Could you check a few things on this model? Use its own coordinates, in mm. Face numbers are marked on the shaded views. A direction names the side the tool comes from. Round coordinates to 2 decimals unless told otherwise and drop trailing zeros. Write each loop counter-clockwise with the first axis right and the second up, starting at its lowest first coordinate (ties: lowest second). Pieces come first, ordered by that corner, then holes. Notation, with made-up numbers: M 7.25,14 L 52.25,14 A20 ccw 52.25,51 Z; hole C -26,-4.5 d10. An arc over 180 degrees is marked long. One line per question, with ' | ' between items. Start each with the question number.
```python
from build123d import *

# Parameters (mm, degrees)
SKETCH4_R           = 3.175
SKETCH4_R_2         = 3.96875
SKETCH4_R_3         = 5.1
SKETCH4_R_4         = 1.6
SKETCH4_R_5         = 2
BOSS_EXTRUDE2_DEPTH = 6.35


with BuildPart() as part:
    # Sketch4 → Boss-Extrude2 (new body)
    with BuildSketch(Plane(origin=(0, 0, 0), x_dir=(1, 0, 0), z_dir=(0, 1, 0))):
        with BuildLine():
            Line((40.257702493, -18.4375), (21.46596982, -18.4375))
            ThreePointArc((21.46596982, -18.4375), (19.855794242, -18.080532669), (18.547340491, -17.076520793))
            Line((18.547340491, -17.076520793), (9.268629328, -6.01858343))
            ThreePointArc((9.268629328, -6.01858343), (6.86044471, -4.691952465), (4.186444468, -5.331503545))
            Line((4.186444468, -5.331503545), (-15.327970397, -18.794247435))
            ThreePointArc((-15.327970397, -18.794247435), (-21.058470009, -18.050117151), (-20.917416467, -12.27322702))
            Line((-20.917416467, -12.27322702), (-8.5725, 0.781747009))
            Line((-8.5725, 0.781747009), (-8.5725, 26.9875))
            ThreePointArc((-8.5725, 26.9875), (-7.456576836, 29.681576836), (-4.7625, 30.7975))
            Line((-4.7625, 30.7975), (52.3875, 30.7975))
            ThreePointArc((52.3875, 30.7975), (55.081576836, 29.681576836), (56.1975, 26.9875))
            Line((56.1975, 26.9875), (56.1975, 19.362095927))
            ThreePointArc((56.1975, 19.362095927), (55.797199918, 17.662082259), (54.680415238, 16.319294633))
            Line((54.680415238, 16.319294633), (48.985566477, 12.027918285))
            ThreePointArc((48.985566477, 12.027918285), (47.868781798, 10.685130659), (47.468481715, 8.985116992))
            Line((47.468481715, 8.985116992), (47.468481715, -10.980610773))
            ThreePointArc((47.468481715, -10.980610773), (47.203372649, -12.376980446), (46.444939319, -13.579024524))
            Line((46.444939319, -13.579024524), (43.044160097, -17.225913752))
            ThreePointArc((43.044160097, -17.225913752), (41.776936446, -18.121498883), (40.257702493, -18.4375))
        make_face()
        with Locations(Location((0, 0, 0), (0, 0, 270))):
            Circle(SKETCH4_R, mode=Mode.SUBTRACT)
        with Locations(Location((-1.5875, 21.9075, 0), (0, 0, 270))):
            Circle(SKETCH4_R_2, mode=Mode.SUBTRACT)
        with Locations(Location((49.2125, 21.9075, 0), (0, 0, 270))):
            Circle(SKETCH4_R_2, mode=Mode.SUBTRACT)
        with Locations(Location((39.848481715, -4.1275, 0), (0, 0, 270))):
            Circle(SKETCH4_R_3, mode=Mode.SUBTRACT)
        with Locations(Location((39.848481715, -14.6275, 0), (0, 0, 270))):
            Circle(SKETCH4_R_4, mode=Mode.SUBTRACT)
        with Locations(Location((39.848481715, 6.3725, 0), (0, 0, 270))):
            Circle(SKETCH4_R_4, mode=Mode.SUBTRACT)
        with Locations(Location((24.012521227, -14.703599027, 0), (0, 0, 270))):
            Circle(SKETCH4_R_5, mode=Mode.SUBTRACT)
        with Locations(Location((-17.78, -15.24, 0), (0, 0, 270))):
            Circle(SKETCH4_R_5, mode=Mode.SUBTRACT)
        with BuildLine():
            Line((40.3225, 26.9875), (40.3225, 16.611657969))
            ThreePointArc((40.3225, 16.611657969), (40.174907062, 15.561479644), (39.743563246, 14.592665573))
            Line((39.743563246, 14.592665573), (31.537418469, 1.460088735))
            ThreePointArc((31.537418469, 1.460088735), (31.106074654, 0.491274664), (30.958481715, -0.558903662))
            Line((30.958481715, -0.558903662), (30.958481715, -3.507298313))
            ThreePointArc((30.958481715, -3.507298313), (29.842558552, -6.20137515), (27.148481715, -7.317298313))
            Line((27.148481715, -7.317298313), (18.766481715, -7.317298313))
            ThreePointArc((18.766481715, -7.317298313), (17.156306138, -6.960330982), (15.847852387, -5.956319106))
            Line((15.847852387, -5.956319106), (8.193870672, 3.165341101))
            ThreePointArc((8.193870672, 3.165341101), (7.532271115, 4.311265148), (7.3025, 5.614361894))
            Line((7.3025, 5.614361894), (7.3025, 26.9875))
            Line((7.3025, 26.9875), (40.3225, 26.9875))
        make_face(mode=Mode.SUBTRACT)
        with BuildLine():
            Line((-13.417009712, -14.390093684), (-4.038317295, -7.919854381))
            ThreePointArc((-4.038317295, -7.919854381), (-6.749791195, -5.78553531), (-8.444304622, -2.779535833))
            Line((-8.444304622, -2.779535833), (-16.272811714, -11.058324681))
            ThreePointArc((-16.272811714, -11.058324681), (-14.405104402, -12.347232345), (-13.417009712, -14.390093684))
        make_face(mode=Mode.SUBTRACT)
        with BuildLine():
            Line((2.2225, 7.28868258), (2.2225, 15.308386423))
            ThreePointArc((2.2225, 15.308386423), (-1.965402874, 14.296876542), (-6.0325, 15.718285591))
            Line((-6.0325, 15.718285591), (-6.0325, 4.65546386))
            ThreePointArc((-6.0325, 4.65546386), (-2.315704041, 7.259608446), (2.2225, 7.28868258))
        make_face(mode=Mode.SUBTRACT)
    extrude(amount=-BOSS_EXTRUDE2_DEPTH)


solid = part.part
```
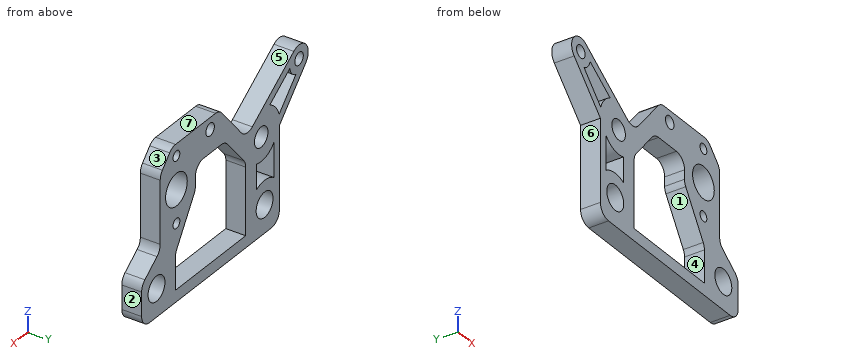
1. Which directions (+Z, -Z, +X, -X, +Y, -Y) give clear straight access to the entire face, cutting with the end or side of a thin tool? Please do the marked faces 4, 5, 6 and 7.
2. I'm going to push flat-ended pins straight in: P1, Ø2.5, axis at y = -2, z = 2.5, coming from the -X side; P2, Ø1, axis at y = -3.5, z = -10, coming from the +X side; P3, Ø3, axis at y = -3, z = -11.5, coming from the -X side. Where does each tip first touch, or does it pass through?
3. I need wall thicknesses on line 1 along X through (y, z) = (-3, -25); line 2 along X through (y, z) = (-3.5, -6); line 3 along Z through (x, y) = (-2, -4.75). Which ranges of each line are inside material? Lowest first, please. Write a range as from..to.
4. Suppose I cut it at C-C (x = 0). Count the separate pieces of the cut face and the enclosed holes in it, and give its area (3 significant figures).
5. If we mould it in two halves opening along Z, with no side actions, what happens to the marked faces 1, 2 and 3? For each: released by +Z, released by -Z, zero draft, split by the parting line, or undercut.
6. Suppose I cut it at B-B (x = -17.78). Write out the boundary of the cut face in (y, z), and give its area (3 significant figures).
7. Suppose I cut it at A-A (z = 15.24). Write out the boundary of the cut face in (x, y), and give its area (3 significant figures).
Computed:
1) face 4: +Y, -Y | face 5: +Z, +Y, -Y | face 6: -Z, -X, +Y, -Y | face 7: +Z, +X, +Y, -Y
2) P1: stops at x = -12.86 | P2: stops at x = 47.78 | P3: stops at x = -8.57
3) line 1: x = -8.57..-4.07, 0.9..7.3, 40.32..46.73, 51.7..56.2 | line 2: x = -8.57..-6.03, -4.7..7.3, 34.37..38.29, 41.4..47.47 | line 3: z = -30.8..-25.85, -17.96..-14.3, -7.35..-2.47, 2.47..9.6
4) separate pieces: 4 | enclosed holes: 0 | area: 118 mm²
5) face 1: undercut | face 2: zero draft | face 3: released by +Z
6) outline: M -6.35,8.96 L 0,8.96 L 0,13.24 L -6.35,13.24 Z; M -6.35,17.24 L 0,17.24 L 0,19.56 L -6.35,19.56 Z | area: 41.9 mm²
7) outline: M -22.1,-6.35 L -19.78,-6.35 L -19.78,0 L -22.1,0 Z; M -15.78,-6.35 L -10.18,-6.35 L -10.18,0 L -15.78,0 Z; M 17.01,-6.35 L 22.09,-6.35 L 22.09,0 L 17.01,0 Z; M 25.94,-6.35 L 38.37,-6.35 L 38.37,0 L 25.94,0 Z; M 41.33,-6.35 L 44.9,-6.35 L 44.9,0 L 41.33,0 Z | area: 184 mm²
